Verification items for the finished model (mm, model axes). Round coordinates to 2 decimals unless told otherwise and drop trailing zeros. Write each loop counter-clockwise with the first axis right and the second up, starting at its lowest first coordinate (ties: lowest second). Pieces come first, ordered by that corner, then holes. Notation, with made-up numbers: M 61,-34 L 101,-34 A30 cw 101,-11 Z; hole C 84,47 d2. An arc over 180 degrees is marked long. One line per question, with ' | ' between items.
from build123d import *

# Parameters (mm, degrees)
SKETCH1_R           = 23.5
BOSS_EXTRUDE1_DEPTH = 2
SKETCH2_R           = 1
SKETCH2_R_2         = 1.25
CUT_EXTRUDE1_DEPTH  = 34.294143629
CUT_EXTRUDE2_REACH  = 35.294
SKETCH3_R           = 4


with BuildPart() as part:
    # Sketch1 → Boss-Extrude1 (new body)
    with BuildSketch(Plane(origin=(0, 0, 0), x_dir=(1, 0, 0), z_dir=(0, 1, 0))):
        with Locations(Location((0, 0, 0), (0, 0, 270))):
            Circle(SKETCH1_R)
    extrude(amount=BOSS_EXTRUDE1_DEPTH)

    # Sketch2 → Cut-Extrude1 (cut, through all)
    with BuildSketch(Plane(origin=(0, 2, 0), x_dir=(1, 0, 0), z_dir=(0, 1, 0))):
        with Locations(Location((0, 8.227062517, 0), (0, 0, 270))):
            Circle(SKETCH2_R)
        with Locations(Location((8.227062517, 0, 0), (0, 0, 270))):
            Circle(SKETCH2_R)
        with Locations(Location((0, -8.227062517, 0), (0, 0, 270))):
            Circle(SKETCH2_R)
        with Locations(Location((-8.227062517, 0, 0), (0, 0, 270))):
            Circle(SKETCH2_R)
        with Locations(Location((0, 19, 0), (0, 0, 270))):
            Circle(SKETCH2_R_2)
        with Locations(Location((16.454482672, -9.5, 0), (0, 0, 270))):
            Circle(SKETCH2_R_2)
        with Locations(Location((-16.454482672, -9.5, 0), (0, 0, 270))):
            Circle(SKETCH2_R_2)
    extrude(amount=-CUT_EXTRUDE1_DEPTH, mode=Mode.SUBTRACT)

    # Sketch3 → Cut-Extrude2 (cut, up to next)
    with BuildSketch(Plane.XZ, mode=Mode.PRIVATE) as cut_extrude2_sk1:
        with Locations(Location((0, 0, 0), (0, 0, 270))):
            Circle(SKETCH3_R)
    cut_extrude2_tool1 = extrude(cut_extrude2_sk1.sketch, amount=-CUT_EXTRUDE2_REACH, mode=Mode.PRIVATE) & part.part
    add(cut_extrude2_tool1.solids().sort_by_distance((0, 0, 0))[0], mode=Mode.SUBTRACT)


solid = part.part
1. Mould release check, pull along X, two halves, no side actions. Record for faces 1 (the face through (-9.203, 1.014, -0.217)), 2 (the face through (-5, 0, 0)), 3 (the face through (15.88, 0.99, -17.32)): pulls with the +X half, pulls with the -X half, needs draft (parallel to the pull), parting line crosses it, or undercut.
Results:
face 1: undercut | face 2: needs draft | face 3: parting line crosses it
2. Section check D-D, the plane y = 0.45. Count the separate pieces of the cut face and the enclosed holes in it, then the cut area to 3 significant figures.
Results:
separate pieces: 1 | enclosed holes: 8 | area: 1,660 mm2
3. Section check A-A, the plane x = 0. Record the cut outline in (y, z), then the cut area to 3 significant figures.
Results:
outline: M 0,-23.5 L 2,-23.5 L 2,-20.25 L 0,-20.25 Z; M 0,-17.75 L 2,-17.75 L 2,-9.23 L 0,-9.23 Z; M 0,-7.23 L 2,-7.23 L 2,-4 L 0,-4 Z; M 0,4 L 2,4 L 2,7.23 L 0,7.23 Z; M 0,9.23 L 2,9.23 L 2,23.5 L 0,23.5 Z | area: 65.0 mm2
4. Thickness scan on line 1 (X direction, y = 0.85, z = 0); line 2 (Z direction, x = 0.5, y = 1.75); line 3 (Z direction, x = 17.5, y = 1). Record the ranges inside material, lowest first.
Results:
line 1: x = -23.5 to -9.23, -7.23 to -4, 4 to 7.23, 9.23 to 23.5 | line 2: z = -23.49 to -20.15, -17.85 to -9.09, -7.36 to -3.97, 3.97 to 7.36, 9.09 to 23.49 | line 3: z = -15.68 to 8.81, 10.19 to 15.68
5. Section check C-C, the plane z = -19. Record the cut outline in (x, y).
Results:
outline: M -13.83,0 L -1.25,0 L -1.25,2 L -13.83,2 Z; M 1.25,0 L 13.83,0 L 13.83,2 L 1.25,2 Z
6. Go/stop test with a flat-tipped pin: P1, Ø1.5, axis at x = 0, z = -19, coming from the +Y side. Record where the tip stops, or that it passes through.
Results:
P1: passes through
7. Section check B-B, the plane z = 0. Record the cut outline in (x, y).
Results:
outline: M -23.5,0 L -9.23,0 L -9.23,2 L -23.5,2 Z; M -7.23,0 L -4,0 L -4,2 L -7.23,2 Z; M 4,0 L 7.23,0 L 7.23,2 L 4,2 Z; M 9.23,0 L 23.5,0 L 23.5,2 L 9.23,2 Z
